from build123d import *

# Parameters (mm, degrees)
BOSS_EXTRUDE1_DEPTH = 30
SKETCH2_W           = 5
SKETCH2_H           = 22
CUT_EXTRUDE1_DEPTH  = 77
SKETCH3_W           = 35
SKETCH3_H           = 3
BOSS_EXTRUDE2_DEPTH = 10


with BuildPart() as part:
    # Sketch1 → Boss-Extrude1 (new body)
    with BuildSketch(Plane.XY):
        Polygon((-48, 3), (48, 3), (48, 0), (28, 0), (28, -22), (25, -22), (25, 0), (-25, 0), (-25, -22), (-28, -22), (-28, 0), (-48, 0), align=None)
    extrude(amount=BOSS_EXTRUDE1_DEPTH)

    # Sketch2 → Cut-Extrude1 (cut, through all)
    with BuildSketch(Plane.ZY.offset(28)):
        with Locations((2.5, -11)):
            Rectangle(SKETCH2_W, SKETCH2_H)
        with Locations((27.5, -11)):
            Rectangle(SKETCH2_W, SKETCH2_H)
    extrude(amount=-CUT_EXTRUDE1_DEPTH, mode=Mode.SUBTRACT)

    # Sketch3 → Boss-Extrude2 (add)
    with BuildSketch(Plane(origin=(0, 3, 0), x_dir=(1, 0, 0), z_dir=(0, 1, 0))):
        with Locations((0, -15)):
            Rectangle(SKETCH3_W, SKETCH3_H)
    extrude(amount=BOSS_EXTRUDE2_DEPTH)


solid = part.part
Read the model definition and answer for the solid it produces. Units are mm, in the model's axes. A direction names the side the tool comes from. Round coordinates to 2 decimals unless told otherwise and drop trailing zeros. Order: outer loops, then holes, each group sorted by start corner. A loop starts at its lowest first (then second) coordinate and runs counter-clockwise, first axis right, second up. Notation, with made-up numbers: (61, 10) - (93, 10) arc R10 cw to (93, 23) - close; hole circle Ø9 at (16, 78). An arc over 180 degrees is marked (long way). Use one line per item in the form item = value. Start each with the question number.
(1) Find the intervals of material crossed by line 1 along X through (y, z) = (-15.5, 23.5); line 2 along Z through (x, y) = (-13, 10); line 3 along Y through (x, z) = (-3, 27), in increasing order. Write a range as from..to.
(2) For faces 1 (the face through (26, -11, 25)), 2 (the face through (0, 8, 13.5)), 3 (the face through (-17.5, 8, 15)), 4 (the face through (28, -11, 15)), determine the directions among +Z, -Z, +X, -X, +Y, -Y from which every point of the face is accessible in a straight line to the end or side of a thin tool.
(3) The part is cut by section C-C (x = -4). Give the vertices of the cut face in (y, z).
(4) Flat-ended cylindrical pins translate along their axes: pin 1 Ø1.5 at (x, y) = (26.5, -8) entering from -Z; pin 2 Ø6 at (x, y) = (-18.5, 3.5) entering from -Z; pin 3 Ø3.5 at (y, z) = (6, 15) entering from -X; pin 4 Ø10 at (y, z) = (-6, 18.5) entering from +X. Find the tip coordinate at first contact, or state that the pin passes through.
(5) Determine the mould class of faces 5 (the face through (25, -11, 15)), 6 (the face through (-27, -11, 5)), 7 (the face through (17.5, 8, 15)) for opening direction X: +X half, -X half, draft (parallel to the pull), parting line (faces both ways), or undercut.
(6) The part is cut by section B-B (z = 20.75). Give the vertices of the cut face in (x, y), then the cut area to 3 significant figures.
(7) The part is cut by section A-A (y = -13). Give the vertices of the cut face in (x, z).
(8) The part is cut by section D-D (y = 5.5). Give the vertices of the cut face in (x, z).
Checked values:
q1.line_1 = -28..-25, 25..28
q1.line_2 = 13.5..16.5
q1.line_3 = 0..3
q2.face_1 = +Z, +X, -X, -Y
q2.face_2 = -Z, +X, -X, +Y
q2.face_3 = +Z, -Z, -X, +Y
q2.face_4 = +Z, -Z, +X, -Y
q3.outline = (0, 0) - (3, 0) - (3, 13.5) - (13, 13.5) - (13, 16.5) - (3, 16.5) - (3, 30) - (0, 30) - close
q4.pin_1 = 5
q4.pin_2 = 0
q4.pin_3 = -17.5
q4.pin_4 = 28
q5.face_5 = undercut
q5.face_6 = draft
q5.face_7 = +X half
q6.outline = (-48, 0) - (-28, 0) - (-28, -22) - (-25, -22) - (-25, 0) - (25, 0) - (25, -22) - (28, -22) - (28, 0) - (48, 0) - (48, 3) - (-48, 3) - close
q6.area = 420 mm^2
q7.outline = (-28, 5) - (-25, 5) - (-25, 25) - (-28, 25) - close; (25, 5) - (28, 5) - (28, 25) - (25, 25) - close
q8.outline = (-17.5, 13.5) - (17.5, 13.5) - (17.5, 16.5) - (-17.5, 16.5) - close
